```python
from build123d import *

# Parameters (mm, degrees)
SKETCH1_W          = 76.2
SKETCH1_H          = 19.0246
CHAMFER1_SIZE      = 2.286
CUT_EXTRUDE2_START = -38.1
SKETCH2_W          = 26.9748
SKETCH2_H          = 266.7
CUT_EXTRUDE2_DEPTH = 19.05


with BuildPart() as part:
    # Sketch1 → Revolve1 (revolve)
    with BuildSketch(Plane(origin=(0, 0, 0), x_dir=(0, 1, 0), z_dir=(0, 0, 1)), mode=Mode.PRIVATE) as revolve1_sk:
        with Locations((0, 123.8377)):
            Rectangle(SKETCH1_W, SKETCH1_H)
    revolve(revolve1_sk.sketch.rotate(Axis((0, -63.5, 0), (0, 1, 0)), 270), axis=Axis((0, -63.5, 0), (0, 1, 0)))

    # Chamfer1
    chamfer1_edges = [part.edges().sort_by_distance(p)[0] for p in [
        (0, -38.1, 114.3254),
        (0, 38.1, 114.3254),
    ]]
    chamfer(chamfer1_edges, length=CHAMFER1_SIZE)

    # Sketch2 → Cut-Extrude2 (cut)
    with BuildSketch(Plane(origin=(0, 0, 0), x_dir=(-1, 0, 0), z_dir=(0, 1, 0)).offset(CUT_EXTRUDE2_START)):
        with Locations((0, 133.35)):
            Rectangle(SKETCH2_W, SKETCH2_H)
    extrude(amount=CUT_EXTRUDE2_DEPTH, mode=Mode.SUBTRACT)


solid = part.part
```
Read the model definition and answer for the solid it produces. Units are mm, in the model's axes. A direction names the side the tool comes from. Give positions to 0.01 mm unless a question says otherwise; leave off trailing zeros. Write each loop counter-clockwise with the first axis right and the second up, starting at its lowest first coordinate (ties: lowest second). Pieces come first, ordered by that corner, then holes. Notation, with made-up numbers: (86, 20) -> (95, 20) arc R19 ccw to (95, 27) -> close; hole circle Ø2 at (-29, -18.75). An arc over 180 degrees is marked (long way). Answer as a JSON object with one key per item and string values.
1) For a pull along Z with two mould halves and no side action, classify faces 3 (the cylindrical face through (-40.055, 0.533, -127.192)), 4 (the flat face through (0, -19.05, 124)), 5 (the cylindrical face through (43.787, 0.501, -105.608)) as pulls with the +Z half, pulls with the -Z half, needs draft (parallel to the pull), parting line crosses it, or undercut.
Findings below:
{"face 3": "parting line crosses it", "face 4": "needs draft", "face 5": "undercut"}
2) Straight lines are drawn through the part: probe 1 along X at (y, z) = (21, 0); probe 2 along Z at (x, y) = (4, 10); probe 3 along Z at (x, y) = (-11.5, 2.5). For each, find the intervals that lie inside material, in ascending order. Write a range as from..to.
Findings below:
{"probe 1": "x = -133.35..-114.33, 114.33..133.35", "probe 2": "z = -133.29..-114.26, 114.26..133.29", "probe 3": "z = -132.85..-113.75, 113.75..132.85"}
3) A tool of negligible diameter and unlimited length cuts with its end or side. For faces 1 (the conical face through (101.553, 35.957, -52.82)), 2 (the flat face through (-13.487, -29, 123)), from which of +Z, -Z, +X, -X, +Y, -Y can it reach the whole face along a straight path? Write none if from no direction.
Findings below:
{"face 1": "+Y", "face 2": "+Z, -Y"}
4) Flat-ended cylindrical pins translate along their axes: pin 1 Ø4 at (x, y) = (-61, -2.5) entering from -Z; pin 2 Ø1 at (y, z) = (-12, -25) entering from -X; pin 3 Ø2 at (x, y) = (-88, 7.5) entering from +Z. Find the tip coordinate at first contact, or state that the pin passes through.
Findings below:
{"pin 1": "stops at z = -119.59", "pin 2": "stops at x = -131.08", "pin 3": "stops at z = 101.06"}
5) Section B-B on y = 0 is taken. Write down the section's boundary in (x, z), then the cut area to 3 significant figures.
Findings below:
{"outline": "circle Ø266.7 at (0, 0); hole circle Ø228.65 at (0, 0)", "area": "14,800 mm^2"}
6) Section A-A on z = 0 is taken. Write down the section's boundary in (x, y), then the cut area to 3 significant figures.
Findings below:
{"outline": "(-133.35, -38.1) -> (-116.61, -38.1) -> (-114.33, -35.81) -> (-114.33, 35.81) -> (-116.61, 38.1) -> (-133.35, 38.1) -> close; (114.33, -35.81) -> (116.61, -38.1) -> (133.35, -38.1) -> (133.35, 38.1) -> (116.61, 38.1) -> (114.33, 35.81) -> close", "area": "2,890 mm^2"}
